```python
from build123d import *

# Parameters (mm, degrees)
SKETCH1_R           = 22.5
SKETCH1_R_2         = 20
BOSS_EXTRUDE1_DEPTH = 5
SKETCH4_R           = 2.5
BOSS_EXTRUDE3_DEPTH = 30
SKETCH5_R           = 20
CUT_EXTRUDE1_DEPTH  = 39.810436902
CIRPATTERN1_COUNT   = 8
SKETCH6_R           = 20
CUT_EXTRUDE2_DEPTH  = 44.588989596
SKETCH7_OUTSIDE_W   = 79.088
SKETCH7_OUTSIDE_H   = 79.088
SKETCH7_OUTSIDE_R   = 30
CUT_EXTRUDE4_DEPTH  = 44.588989596


with BuildPart() as part:
    # Sketch1 → Boss-Extrude1 (new, symmetric)
    with BuildSketch(Plane(origin=(0, 0, 0), x_dir=(1, 0, 0), z_dir=(0, 1, 0))):
        with Locations(Location((0, 0, 0), (0, 0, 270))):
            Circle(SKETCH1_R)
        with Locations(Location((0, 0, 0), (0, 0, 270))):
            Circle(SKETCH1_R_2, mode=Mode.SUBTRACT)
    extrude(amount=BOSS_EXTRUDE1_DEPTH, both=True)

    # Sketch4 → Boss-Extrude3 (add)
    with BuildSketch(Plane(origin=(0, 0, 0), x_dir=(0, 0, -1), z_dir=(1, 0, 0))):
        with Locations(Location((0, 0, 0), (0, 0, 180))):
            Circle(SKETCH4_R)
    boss_extrude3 = extrude(amount=BOSS_EXTRUDE3_DEPTH)

    # Sketch5 → Cut-Extrude1 (cut, through all)
    with BuildSketch(Plane.XZ.offset(5)):
        with Locations(Location((0, 0, 0), (0, 0, 90))):
            Circle(SKETCH5_R)
    extrude(amount=-CUT_EXTRUDE1_DEPTH, mode=Mode.SUBTRACT)

    # CirPattern1: Boss-Extrude3 ×8 about axis
    cirpattern1_axis = Axis((0, 0, 0), (0, 1, 0))
    for i in range(1, CIRPATTERN1_COUNT):
        add(boss_extrude3.rotate(cirpattern1_axis, i * 360 / CIRPATTERN1_COUNT))

    # Sketch6 → Cut-Extrude2 (cut, through all)
    with BuildSketch(Plane.XZ.offset(5)):
        with Locations(Location((0, 0, 0), (0, 0, 90))):
            Circle(SKETCH6_R)
    extrude(amount=-CUT_EXTRUDE2_DEPTH, mode=Mode.SUBTRACT)

    # Sketch7 outside → Cut-Extrude4 (cut, through all)
    with BuildSketch(Plane(origin=(0, 5, 0), x_dir=(1, 0, 0), z_dir=(0, 1, 0))):
        Rectangle(SKETCH7_OUTSIDE_W, SKETCH7_OUTSIDE_H)
        Circle(SKETCH7_OUTSIDE_R, mode=Mode.SUBTRACT)
    extrude(amount=-CUT_EXTRUDE4_DEPTH, mode=Mode.SUBTRACT)


solid = part.part
```
Build history of the part. All positions in model axes, mm. A direction names the side the tool comes from. Round coordinates to 2 decimals unless told otherwise and drop trailing zeros. Order: outer loops, then holes, each group sorted by start corner. A loop starts at its lowest first (then second) coordinate and runs counter-clockwise, first axis right, second up. Notation, with made-up numbers: (89.25, -37.5) -> (124.25, -37.5) arc R7 ccw to (124.25, -24.5) -> close; hole circle Ø2 at (4, -32). An arc over 180 degrees is marked (long way). Answer in a Markdown table with one row per item.
1) Mould opens along Z. For faces 5 (the cylindrical face through (-8.618, 0.07, 20.784)), 6 (the cylindrical face through (20.24, -0.11, 16.71)), 7 (the cylindrical face through (-30, 0, 0)), 8 (the cylindrical face through (0, 0, 30)) say: released by +Z, released by -Z, zero draft, split by the parting line, or undercut.
Values:
| item | result |
|---|---|
| face 5 | undercut |
| face 6 | undercut |
| face 7 | split by the parting line |
| face 8 | released by +Z |
2) Pin check, flat tips, straight feed: P1, Ø6, axis at y = 0, z = -7, coming from the +X side; P2, Ø2, axis at y = 2, z = 18.5, coming from the +X side; P3, Ø2, axis at x = 9, y = -1.5, coming from the +Z side. Stop position of each tip, or through.
Values:
| item | result |
|---|---|
| P1 | x = 22.14 |
| P2 | x = 22.24 |
| P3 | z = 21.03 |
3) Band-saw the part on A-A on z = 0. Give the cut face in (x, y).
Values:
| item | result |
|---|---|
| outline | (-30, -2.5) -> (-22.5, -2.5) -> (-22.5, -5) -> (-20, -5) -> (-20, 5) -> (-22.5, 5) -> (-22.5, 2.5) -> (-30, 2.5) -> close; (20, -5) -> (22.5, -5) -> (22.5, -2.5) -> (30, -2.5) -> (30, 2.5) -> (22.5, 2.5) -> (22.5, 5) -> (20, 5) -> close |
4) Wall check: L1, parallel to Z at x = -0.5, y = 2; L2, parallel to X at y = -0.75, z = 0; L3, parallel to Z at x = -1, y = -3. Give the ranges that are in metal, low to high.
Values:
| item | result |
|---|---|
| L1 | -30 to -19.99, 19.99 to 30 |
| L2 | -30 to -20, 20 to 30 |
| L3 | -22.48 to -19.97, 19.97 to 22.48 |
5) Band-saw the part on C-C on z = -25.5. Give the cut face in (x, y), and give its area (3 significant figures).
Values:
| item | result |
|---|---|
| outline | circle Ø5 at (0, 0) |
| area | 19.6 mm2 |
6) Which spindle directions (+Z, -Z, +X, -X, +Y, -Y) get a long thin tool onto all of the face, cutting with end or side? Do faces 1 (the cylindrical face through (-2.5, -0.1, -26.1)), 2 (the cylindrical face through (-26.1, 1.5, 2)), 3 (the cylindrical face through (26.1, -0.1, -2.5)), 4 (the cylindrical face through (2, 1.5, 26.1)). Say none if no direction does.
Values:
| item | result |
|---|---|
| face 1 | -Z |
| face 2 | -X |
| face 3 | +X |
| face 4 | +Z |
7) Band-saw the part on D-D on z = 11. Give the cut face in (x, y), and give its area (3 significant figures).
Values:
| item | result |
|---|---|
| outline | (-19.63, -5) -> (-16.7, -5) -> (-16.7, 5) -> (-19.63, 5) -> close; (16.7, -5) -> (19.63, -5) -> (19.63, 5) -> (16.7, 5) -> close |
| area | 58.5 mm2 |
